```python
from build123d import *

# Parameters (mm, degrees)
ESQUISSE1_W                  = 25
ESQUISSE1_H                  = 45
ESQUISSE1_R                  = 1.863501178
ESQUISSE1_R_2                = 1.93430269
ESQUISSE1_R_3                = 1.939737899
ESQUISSE1_R_4                = 1.854627201
BOSS_EXTRU_1_DEPTH           = 3
BOSS_EXTRU_2_DEPTH           = 10
ENL_V_MAT_EXTRU_1_DEPTH      = 30.52964612
ENL_V_MAT_EXTRU_1_DEPTH_BACK = 30.52964612
ESQUISSE3_R                  = 1.5
ESQUISSE4_R                  = 1.5
BOSS_EXTRU_3_DEPTH           = 2
CONG_1_R                     = 1
ESQUISSE5_W                  = 14
ESQUISSE5_H                  = 3
ENL_V_MAT_EXTRU_2_DEPTH      = 34.421549934


with BuildPart() as part:
    # Esquisse1 → Boss.-Extru.1 (new body)
    with BuildSketch(Plane.XY):
        Rectangle(ESQUISSE1_W, ESQUISSE1_H)
        with Locations((-7.354431697, -16.736502833)):
            Circle(ESQUISSE1_R, mode=Mode.SUBTRACT)
        with Locations((7.237211302, -16.593743463)):
            Circle(ESQUISSE1_R_2, mode=Mode.SUBTRACT)
        with Locations((-7.142905367, 18.055953642)):
            Circle(ESQUISSE1_R_3, mode=Mode.SUBTRACT)
        with Locations((7.324743745, 18.008545284)):
            Circle(ESQUISSE1_R_4, mode=Mode.SUBTRACT)
    extrude(amount=BOSS_EXTRU_1_DEPTH)

    # Esquisse2 → Boss.-Extru.2 (add)
    with BuildSketch(Plane.XY):
        Polygon((7, -22.5), (7, -24), (14, -24), (14, 24), (-14, 24), (-14, -24), (-7, -24), (-7, -22.5), (-12.5, -22.5), (-12.5, 22.5), (12.5, 22.5), (12.5, -22.5), align=None)
    extrude(amount=BOSS_EXTRU_2_DEPTH)

    # Esquisse3 → Enlèv. mat.-Extru.1 (cut, two sides: drawn at the far end of the back side and taken through both)
    with BuildSketch(Plane(origin=(0, 0, 0), x_dir=(0, 0, -1), z_dir=(1, 0, 0)).offset(-ENL_V_MAT_EXTRU_1_DEPTH_BACK)):
        with Locations((-7, -14)):
            Circle(ESQUISSE3_R)
    extrude(amount=ENL_V_MAT_EXTRU_1_DEPTH + ENL_V_MAT_EXTRU_1_DEPTH_BACK, mode=Mode.SUBTRACT)

    # Esquisse4 → Boss.-Extru.3 (add)
    # profile 1 of 2: a face of its own
    with BuildSketch(Plane.XY):
        with BuildLine():
            Line((-14, 3), (-18, 3))
            ThreePointArc((-18, 3), (-21, 0), (-18, -3))
            Line((-18, -3), (-14, -3))
            Line((-14, -3), (-14, 3))
        make_face()
        with Locations((-18, 0)):
            Circle(ESQUISSE4_R, mode=Mode.SUBTRACT)
    # profile 2 of 2: a face of its own
    with BuildSketch(Plane.XY):
        with BuildLine():
            Line((18, -3), (14, -3))
            Line((14, -3), (14, 3))
            Line((14, 3), (18, 3))
            ThreePointArc((18, 3), (21, 0), (18, -3))
        make_face()
        with Locations(Location((18, 0, 0), (0, 0, 180))):
            Circle(ESQUISSE4_R, mode=Mode.SUBTRACT)
    extrude(amount=BOSS_EXTRU_3_DEPTH)

    # Congé1
    cong_1_edges = [part.edges().sort_by_distance(p)[0] for p in [
        (-14, 0, 2),
        (-14, -3, 1),
        (-14, 3, 1),
        (14, 0, 2),
        (14, 3, 1),
        (14, -3, 1),
    ]]
    fillet(cong_1_edges, radius=CONG_1_R)

    # Esquisse5 → Enlèv. mat.-Extru.2 (cut, through all)
    with BuildSketch(Plane.XY):
        with Locations((0, -21)):
            Rectangle(ESQUISSE5_W, ESQUISSE5_H)
    extrude(amount=ENL_V_MAT_EXTRU_2_DEPTH, mode=Mode.SUBTRACT)


solid = part.part
```
Part model, mm, in its own coordinate system. A direction names the side the tool comes from. Round coordinates to 2 decimals unless told otherwise and drop trailing zeros. Order: outer loops, then holes, each group sorted by start corner. A loop starts at its lowest first (then second) coordinate and runs counter-clockwise, first axis right, second up. Notation, with made-up numbers: M -29,-27 L -8,-27 A16 ccw -8,0 Z; hole C -29,56.5 d11. An arc over 180 degrees is marked long. Put each result on its own line as item: value. Start each with the question number.
1. Slice it at C-C on y = 5. List the corners of the cut face in (x, z), then the cut area to 3 significant figures.
2. Slice it at B-B on y = 0. List the corners of the cut face in (x, z).
3. Drill centre lines: probe 1 along X at (y, z) = (1, 4.5); probe 2 along Y at (x, z) = (11, 5); probe 3 along Y at (x, z) = (-8.5, 1). Where is each one in solid material? Low to high. Write a range as [from, to].
4. Slice it at D-D on x = 1.5. List the corners of the cut face in (y, z), then the cut area to 3 significant figures.
5. Tool access for faces 4 (the face through (-10, -22.5, 6)), 5 (the face through (-16, 0, 2)), 6 (the face through (-17, -3, 1)): list every direction of +Z, -Z, +X, -X, +Y, -Y with a clear straight run to the whole face (end or side of a thin tool).
6. Drop flat-ended pins along their axis: pin 1 (4 mm diameter, centred on y = 12, z = 3.5, fed in from -X); pin 2 (1 mm diameter, centred on x = -4.5, y = -15, fed in from -Z); pin 3 (5 mm diameter, centred on y = -14, z = 7, fed in from +X); pin 4 (2.5 mm diameter, centred on x = 7.24, y = -16.59, fed in from +Z). Give the stop position or say it passes through.
7. Slice it at A-A on z = 7. List the corners of the cut face in (x, y), then the cut area to 3 significant figures.
8. Two-plate mould, pull along Y, no slides. Class faces 1 (the face through (0, 22.5, 6)), 2 (the face through (16, 0, 2)), 3 (the face through (-14.285, -3.301, 1.188)): +Y half, -Y half, draft (parallel to the pull), parting line (faces both ways), or undercut.
Findings:
1. outline: M -14,0 L 14,0 L 14,10 L 12.5,10 L 12.5,3 L -12.5,3 L -12.5,10 L -14,10 Z
1. area: 105 mm2
2. outline: M -21,0 L -19.5,0 L -19.5,2 L -21,2 Z; M -16.5,0 L 16.5,0 L 16.5,2 L 15,2 A1 cw 14,3 L 14,10 L 12.5,10 L 12.5,3 L -12.5,3 L -12.5,10 L -14,10 L -14,3 A1 cw -15,2 L -16.5,2 Z; M 19.5,0 L 21,0 L 21,2 L 19.5,2 Z
3. probe 1: [-14, -12.5], [12.5, 14]
3. probe 2: [-24, -22.5], [22.5, 24]
3. probe 3: [-24, -18.21], [-15.27, 16.67], [19.44, 24]
4. outline: M -19.5,0 L 24,0 L 24,10 L 22.5,10 L 22.5,3 L -19.5,3 Z
4. area: 141 mm2
5. face 4: +Z
5. face 5: +Z, -X, +Y, -Y
5. face 6: +Z, -Z, -X, -Y
6. pin 1: x = -14
6. pin 2: z = 0
6. pin 3: x = 14
6. pin 4: through
7. outline: M -14,-24 L -7,-24 L -7,-22.5 L -12.5,-22.5 L -12.5,-15.5 L -14,-15.5 Z; M -14,-12.5 L -12.5,-12.5 L -12.5,22.5 L 12.5,22.5 L 12.5,-12.5 L 14,-12.5 L 14,24 L -14,24 Z; M 7,-24 L 14,-24 L 14,-15.5 L 12.5,-15.5 L 12.5,-22.5 L 7,-22.5 Z
7. area: 189 mm2
8. face 1: undercut
8. face 2: draft
8. face 3: -Y half
